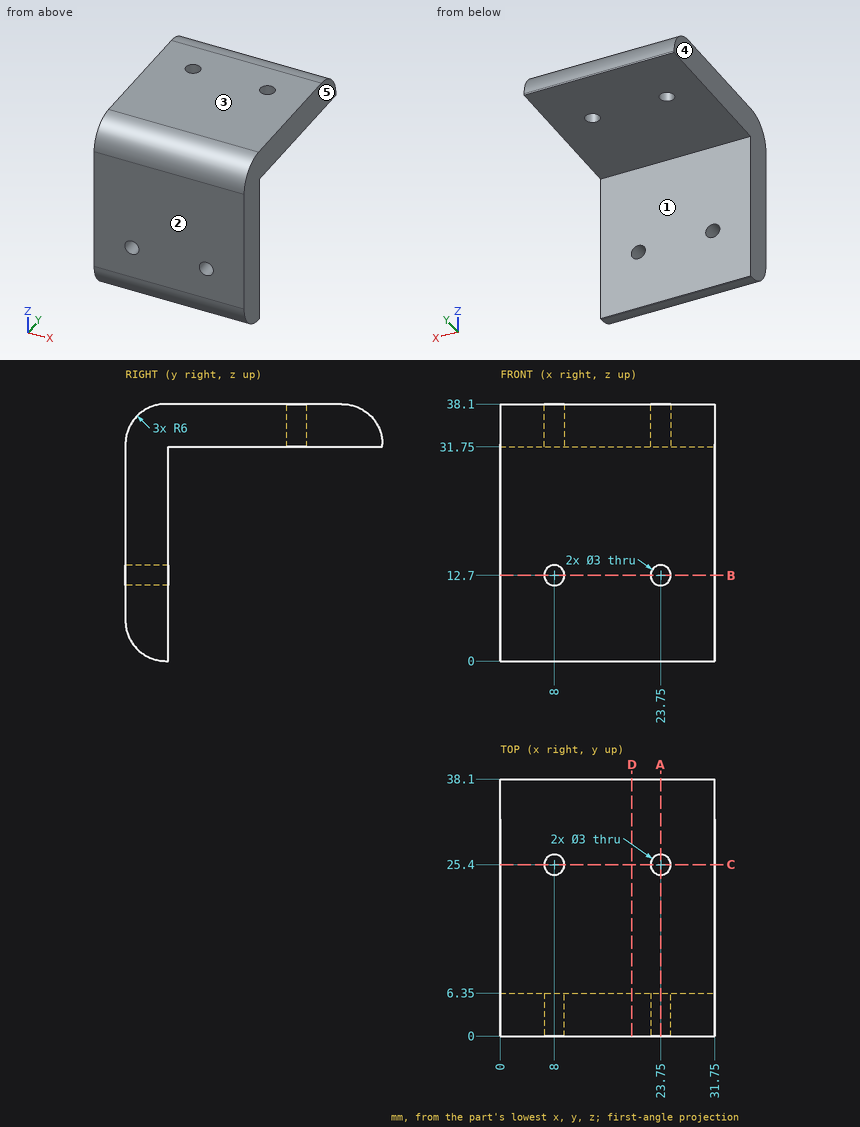
The figure shows three views and two pictorial views of one solid part (mm, origin at its lowest corner). Answer the questions. A direction names the side the tool comes from. Coordinates: 2 decimals unless noted, no trailing zeros. Write each loop counter-clockwise with the first axis right and the second up, starting at its lowest first coordinate (ties: lowest second). Pieces come first, ordered by that corner, then holes. Notation, with made-up numbers: (61, 1) -> (114, 1) arc R25 cw to (114, 30) -> close; hole circle Ø2 at (65.25, 84.25). An arc over 180 degrees is marked (long way). Return JSON: item names as keys, results as strings.
(1) The part is cut by section D-D on x = 19.5. Give the vertices of the cut face in (y, z).
Answers below:
{"outline": "(0, 6) arc R6 ccw to (6, 0) -> (6.35, 0) -> (6.35, 31.75) -> (38.1, 31.75) -> (38.1, 32.1) arc R6 ccw to (32.1, 38.1) -> (6, 38.1) arc R6 ccw to (0, 32.1) -> close"}
(2) Which of the six approach directions +Z, -Z, +X, -X, +Y, -Y give full straight-line access (tool end or side, diameter ignored) to the marked faces 1 and 2?
Answers below:
{"face 1": "-Z, +X, -X, +Y", "face 2": "+Z, -Z, +X, -X, -Y"}
(3) The part is cut by section A-A on x = 23.75. Give the vertices of the cut face in (y, z), then the cut area to 3 significant figures.
Answers below:
{"outline": "(0, 6) arc R6 ccw to (6, 0) -> (6.35, 0) -> (6.35, 11.2) -> (0, 11.2) -> close; (0, 14.2) -> (6.35, 14.2) -> (6.35, 31.75) -> (23.9, 31.75) -> (23.9, 38.1) -> (6, 38.1) arc R6 ccw to (0, 32.1) -> close; (26.9, 31.75) -> (38.1, 31.75) -> (38.1, 32.1) arc R6 ccw to (32.1, 38.1) -> (26.9, 38.1) -> close", "area": "382 mm^2"}
(4) The part is cut by section B-B on z = 12.7. Give the vertices of the cut face in (x, y), then the cut area to 3 significant figures.
Answers below:
{"outline": "(0, 0) -> (6.5, 0) -> (6.5, 6.35) -> (0, 6.35) -> close; (9.5, 0) -> (22.25, 0) -> (22.25, 6.35) -> (9.5, 6.35) -> close; (25.25, 0) -> (31.75, 0) -> (31.75, 6.35) -> (25.25, 6.35) -> close", "area": "164 mm^2"}
(5) The part is cut by section C-C on y = 25.4. Give the vertices of the cut face in (x, z).
Answers below:
{"outline": "(0, 31.75) -> (6.5, 31.75) -> (6.5, 38.1) -> (0, 38.1) -> close; (9.5, 31.75) -> (22.25, 31.75) -> (22.25, 38.1) -> (9.5, 38.1) -> close; (25.25, 31.75) -> (31.75, 31.75) -> (31.75, 38.1) -> (25.25, 38.1) -> close"}
(6) For a pull along X with two mould halves and no side action, classify the marked faces 3, 4 and 5 as pulls with the +X half, pulls with the -X half, needs draft (parallel to the pull), parting line crosses it, or undercut.
Answers below:
{"face 3": "needs draft", "face 4": "pulls with the -X half", "face 5": "pulls with the +X half"}
(7) Each of these flat-tipped pins is pushed along its axis until it touches: P1, Ø9.5, axis at x = 13, z = 9.5, coming from the +Y side; P2, Ø6, axis at x = 27.5, y = 27.5, coming from the -Z side. Where does it stop, or does it pass through?
Answers below:
{"P1": "y = 6.35", "P2": "z = 31.75"}
(8) Consider line 1 along X through (y, z) = (26, 35); line 2 along Z through (x, y) = (20, 20); line 3 along Y through (x, z) = (11.5, 20). Determine where each line is inside the solid, lowest interval first. Write a range as from..to.
Answers below:
{"line 1": "0..6.63, 9.37..22.38, 25.12..31.75", "line 2": "31.75..38.1", "line 3": "0..6.35"}
